Autodesk Inventor part; units mm, degrees
ref_plane "YZ Plane" through (0, 0, 0) normal (1, 0, 0) x (0, 1, 0)
ref_plane "XZ Plane" through (0, 0, 0) normal (0, 1, 0) x (-1, 0, 0)
ref_plane "XY Plane" through (0, 0, 0) normal (0, 0, 1) x (1, 0, 0)
sketch "Sketch1" plane through (0, 0, 0) normal (0, 0, 1) x (1, 0, 0)
  line L0 (0, 0) -> (43.5, 0)
  line L1 (43.5, 0) -> (43.5, 43.5)
  line L2 (43.5, 43.5) -> (0, 43.5)
  line L3 (0, 43.5) -> (0, 0)
  dimension "d0" = 43.5
  dimension "d1" = 43.5
extrude "Extrusion1" add sketch "Sketch1" along normal blind 9
chamfer "Chamfer1" distance 7 angle 45 4 edges at (21.75, 43.5, 9) (0, 21.75, 9) (21.75, 0, 9) (43.5, 21.75, 9)
sketch "Sketch2" plane through (0, 0, 9) normal (0, 0, 1) x (1, 0, 0)
  line L0 (7, 7) -> (36.5, 7)
  line L1 (36.5, 7) -> (36.5, 36.5)
  line L2 (36.5, 36.5) -> (7, 36.5)
  line L3 (7, 36.5) -> (7, 7)
  point P0 (0, 0)
extrude "Extrusion2" add sketch "Sketch2" along normal blind 2
sketch "Sketch3" plane through (36.5, 7, 9) normal (1, 0, 0) x (0, 0, -1)
  line L0 (0, 0) -> (0, 29.5)
  line L1 (-2, 90.75) -> (-2, -61.25)
  line L2 (-23.5, -63.25) -> (-23.5, -53.25)
  line L3 (-23.5, -53.25) -> (-21.5, -53.25)
  line L4 (-21.5, -53.25) -> (-21.5, -61.25)
  line L5 (-21.5, -61.25) -> (-2, -61.25)
  line L6 (-23.5, 92.75) -> (-23.5, 82.75)
  line L7 (-23.5, 82.75) -> (-21.5, 82.75)
  line L8 (-21.5, 82.75) -> (-21.5, 90.75)
  line L9 (-21.5, 90.75) -> (-2, 90.75)
  line L10 (-23.5, -63.25) -> (0, -63.25)
  line L11 (0, -63.25) -> (0, 92.75)
  line L12 (-23.5, 92.75) -> (0, 92.75)
  line L13 (9, -7) -> (9, 36.5)
  dimension "d15" = 10
  dimension "d16" = 2
  dimension "d17" = 8
  dimension "d21" = 156
  dimension "d22" = 23.5
  dimension "d23" = 19.5
  dimension "d24" = 2
  dimension "d27" = 9
  dimension "d28" = 63.25
extrude "Extrusion3" add sketch "Sketch3" against normal blind 29.5
fillet "Fillet1" radius 1 2 edges at (21.75, 36.5, 9) (21.75, 7, 9)
fillet "Fillet2" radius 2 8 edges at (21.75, -56.25, 9) (21.75, 99.75, 9) (21.75, 99.75, 32.5) (21.75, -56.25, 32.5) (21.75, -54.25, 30.5) (21.75, -54.25, 11) (21.75, 97.75, 11) (21.75, 97.75, 30.5)
sketch "Sketch4" plane through (0, 0, 0) normal (0, 0, -1) x (-1, 0, 0)
  line L0 (0, 0) -> (-43.5, 43.5) construction
  line L1 (-38.2071, 38.2071) -> (-43.5, 43.5) construction
  line L2 (-43.5, 43.5) -> (-43.5, 0) construction
  line L3 (-43.5, 0) -> (0, 43.5) construction
  circle A0 centre (-21.75, 21.75) radius 6.625
  dimension "d33" = 13.25
extrude "Extrusion4" cut sketch "Sketch4" against normal blind 8
sketch "Sketch5" plane through (21.75, 21.75, 8) normal (0, 0, -1) x (-1, 0, 0)
  circle A0 centre (0, 0) radius 4
  point P0 (21.75, -21.75)
  dimension "d36" = 8
extrude "Extrusion5" cut sketch "Sketch5" against normal blind 44.75
properties part number "Tripod"
Here's how the part is built. I have some questions about the finished solid (model axes, mm). A direction names the side the tool comes from. Give positions to 0.01 mm unless a question says otherwise; leave off trailing zeros. Write each loop counter-clockwise with the first axis right and the second up, starting at its lowest first coordinate (ties: lowest second). Pieces come first, ordered by that corner, then holes. Notation, with made-up numbers: M -35,55 L -20,55 A29 cw -20,89 Z; hole C 54.25,60.25 d2. An arc over 180 degrees is marked long. Put each result on its own line as item: value. Start each with the question number.
Item 1: On a 3-axis mill with a long thin cutter (end or side, diameter ignored), from which of +Z, -Z, +X, -X, +Y, -Y can I reach the whole of each face in a straight line? I mean faces 1 (the flat face through (17, 22, 8)), 2 (the flat face through (36.5, 22, 10)), 3 (the flat face through (7, 22, 10)), 4 (the flat face through (22, -54.25, 21)). Say none if no direction works.
Item 2: If we section it at D-D, the plane y = 52: Write out the boundary of the cut face in (x, z).
Item 3: Thinking about a two-plate mould opening in Y: for faces 5 (the flat face through (29, 23, 11)), 6 (the flat face through (22, -25, 9)), 7 (the flat face through (22, -56.25, 21)), 8 (the flat face through (21.4, 40.8, 4.7)), which applies, +Y half, -Y half, draft (parallel to the pull), parting line (faces both ways), or undercut?
Item 4: I need wall thicknesses on L1, parallel to Y at x = 29, z = 24.5; L2, parallel to Z at x = 12, y = -30; L3, parallel to Z at x = 13, y = 17. Which ranges of each line are inside material? Lowest first, please. Write a range as from..to.
Item 5: Will these pins go through, and if not, where does the flat tip stop? pin 1 (1 mm diameter, centred on x = 24.5, z = 1, fed in from -Y); pin 2 (17 mm diameter, centred on x = 21.75, y = 21.75, fed in from +Z); pin 3 (3 mm diameter, centred on x = 26.5, y = 93, fed in from -Z); pin 4 (6.5 mm diameter, centred on x = 21.75, y = 21.75, fed in from -Z).
Item 6: If we section it at B-B, the plane y = 21.75: Write out the boundary of the cut face in (x, z) (3 decimals), then the cut area to 4 significant figures.
Item 7: If we section it at C-C, the plane x = 12.5: Write out the boundary of the cut face in (y, z).
Item 8: If we section it at A-A, the plane z = 23: Write out the boundary of the cut face in (x, y).
Values:
1. face 1: -Z
1. face 2: +Z, +X, +Y, -Y
1. face 3: +Z, -X, +Y, -Y
1. face 4: +X, -X
2. outline: M 7,9 L 36.5,9 L 36.5,11 L 7,11 Z
3. face 5: undercut
3. face 6: draft
3. face 7: -Y half
3. face 8: +Y half
4. L1: -56.25..-54.25, 97.75..99.75
4. L2: 9..11
4. L3: 0..11
5. pin 1: y = 0
5. pin 2: z = 11
5. pin 3: z = 9
5. pin 4: through
6. outline: M 0,0 L 15.125,0 L 15.125,8 L 17.75,8 L 17.75,11 L 7,11 L 7,9 L 0,2 Z; M 25.75,8 L 28.375,8 L 28.375,0 L 43.5,0 L 43.5,2 L 36.5,9 L 36.5,11 L 25.75,11 Z
6. area: 271.5 mm²
7. outline: M -56.25,11 A2 ccw -54.25,9 L 4.59,9 A1 cw 5.29,7.29 L 0,2 L 0,0 L 43.5,0 L 43.5,2 L 38.21,7.29 A1 cw 38.91,9 L 97.75,9 A2 ccw 99.75,11 L 99.75,30.5 A2 ccw 97.75,32.5 L 89.75,32.5 L 89.75,30.5 L 95.75,30.5 A2 cw 97.75,28.5 L 97.75,13 A2 cw 95.75,11 L -52.25,11 A2 cw -54.25,13 L -54.25,28.5 A2 cw -52.25,30.5 L -46.25,30.5 L -46.25,32.5 L -54.25,32.5 A2 ccw -56.25,30.5 Z
8. outline: M 7,-56.25 L 36.5,-56.25 L 36.5,-54.25 L 7,-54.25 Z; M 7,97.75 L 36.5,97.75 L 36.5,99.75 L 7,99.75 Z
